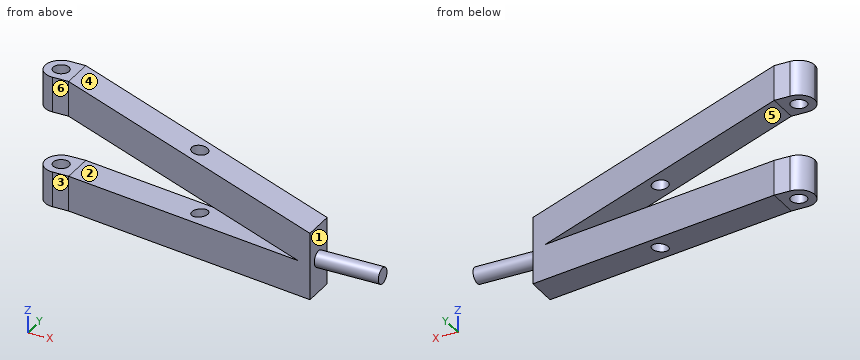
from build123d import *

# Parameters (mm, degrees)
SKETCH10_W              = 27.94
SKETCH10_H              = 25.4
SKETCH12_W              = 27.94
SKETCH12_H              = 25.4
BOSS_EXTRUDE2_DEPTH     = 25.4
SKETCH13_R              = 6.35
CUT_EXTRUDE4_DEPTH      = 105.14
CUT_EXTRUDE5_DEPTH      = 105.14
SKETCH15_R              = 6.35
BOSS_EXTRUDE3_DEPTH     = 50.8
SKETCH16_R              = 6.35
CUT_EXTRUDE6_DEPTH      = 53.07
CUT_EXTRUDE6_DEPTH_BACK = 53.07


with BuildPart() as part:
    # Sweep3: sweep along a curve in space
    with BuildLine() as sweep3_path:
        Line((12.7, 0, 38.1), (241.3, -69.85, 12.7))
    # Sketch10 → Sweep3 (sweep)
    with BuildSketch(Plane(origin=(12.7, 0, 0), x_dir=(0, 0, -1), z_dir=(1, 0, 0))):
        with Locations((-38.1, 0)):
            Rectangle(SKETCH10_W, SKETCH10_H)
    sweep3 = sweep(path=sweep3_path.line)

    # Sketch12 → Boss-Extrude2 (add)
    with BuildSketch(Plane(origin=(12.7, 0, 0), x_dir=(0, 0, -1), z_dir=(1, 0, 0))):
        with Locations((-38.1, 0)):
            Rectangle(SKETCH12_W, SKETCH12_H)
    boss_extrude2 = extrude(amount=-BOSS_EXTRUDE2_DEPTH)

    # Mirror5: Sweep3, Boss-Extrude2 across plane
    add(sweep3.mirror(Plane.XY))
    add(boss_extrude2.mirror(Plane.XY))

    # Sketch13 → Cut-Extrude4 (cut, through all)
    with BuildSketch(Plane(origin=(0, 0, -52.07), x_dir=(-1, 0, 0), z_dir=(0, 0, -1))):
        Circle(SKETCH13_R)
    extrude(amount=-CUT_EXTRUDE4_DEPTH, mode=Mode.SUBTRACT)

    # Sketch14 → Cut-Extrude5 (cut, through all)
    with BuildSketch(Plane(origin=(0, 0, -52.07), x_dir=(-1, 0, 0), z_dir=(0, 0, -1))):
        with BuildLine():
            Line((12.7, 12.7), (0, 12.7))
            ThreePointArc((0, 12.7), (8.980256121, 8.980256121), (12.7, 0))
            Line((12.7, 0), (12.7, 12.7))
        make_face()
    cut_extrude5 = extrude(amount=-CUT_EXTRUDE5_DEPTH, mode=Mode.SUBTRACT)

    # Mirror6: Cut-Extrude5 across plane
    add(cut_extrude5.mirror(Plane.ZX), mode=Mode.SUBTRACT)

    # Sketch15 → Boss-Extrude3 (add)
    with BuildSketch(Plane(origin=(241.3, 0, 0), x_dir=(0, 0, -1), z_dir=(1, 0, 0))):
        with Locations((0, -69.85)):
            Circle(SKETCH15_R)
    extrude(amount=BOSS_EXTRUDE3_DEPTH)

    # Sketch16 → Cut-Extrude6 (cut, two sides)
    with BuildSketch(Plane.XY) as cut_extrude6_sk:
        with Locations((128.524, -34.925)):
            Circle(SKETCH16_R)
    extrude(amount=CUT_EXTRUDE6_DEPTH, mode=Mode.SUBTRACT)
    extrude(cut_extrude6_sk.sketch, amount=-CUT_EXTRUDE6_DEPTH_BACK, mode=Mode.SUBTRACT)


solid = part.part
Check sheet for the modelled part. Datum: model origin and axes. Units: mm. Face numbers are marked on the shaded views. A direction names the side the tool comes from. Round coordinates to 2 decimals unless told otherwise and drop trailing zeros. Loops run counter-clockwise (first coordinate to the right, second up) from the corner with the lowest first, then second, coordinate; pieces in that order, holes last. Notation, with made-up numbers: (-30.5, -31) -> (11.5, -31) arc R23 cw to (11.5, -12) -> close; hole circle Ø8 at (19.5, 38.5). An arc over 180 degrees is marked (long way). Put each result on its own line as item: value. Start each with the question number.
1. Access from +Z, -Z, +X, -X, +Y, -Y to the whole of each face (thin tool, end or side, straight path). Record for the marked faces 1, 2 and 3.
2. Gauge pin test, flat ends, axial feed: pin 1 (16.5 mm diameter, centred on x = 128.524, y = -34.925, fed in from -Z); pin 2 (8 mm diameter, centred on x = 86.5, y = -25.5, fed in from -Z); pin 3 (10 mm diameter, centred on x = 150.5, z = -20, fed in from -Y); pin 4 (20.5 mm diameter, centred on x = 0, y = 0, fed in from -Z). Record the tip position at first contact, or that the pin passes through.
3. Scan lines: probe 1 along Y at (x, z) = (0, -30.5); probe 2 along Z at (x, y) = (139.5, -37); probe 3 along Y at (x, z) = (90, 30.5). Record each from-to range of solid material in increasing order.
4. Section check D-D (y = -69.85). Enter the section's corners in (x, z).
5. Section check A-A (y = -23.5). Enter the section's corners in (x, z), plus the area to 3 significant figures.
6. Draft check along Z on the marked faces 4, 5 and 6. Enter one of: +Z half, -Z half, draft (parallel to the pull), parting line (faces both ways), or undercut.
7. Section check B-B (x = 203.5). Enter the section's corners in (y, z), plus the area to 3 significant figures.
Findings:
1. face 1: +X
1. face 2: -X, +Y, -Y
1. face 3: +Z, -Z, -X, -Y
2. pin 1: stops at z = -40.12
2. pin 2: stops at z = -44.31
2. pin 3: stops at y = -56.33
2. pin 4: stops at z = -52.07
3. probe 1: y = -12.7 to -6.35, 6.35 to 12.7
3. probe 2: z = -37.98 to -10.04, 10.04 to 37.98
3. probe 3: y = -36.32 to -10.92
4. outline: (199.74, -31.29) -> (241.3, -26.67) -> (241.3, -6.35) -> (292.1, -6.35) -> (292.1, 6.35) -> (241.3, 6.35) -> (241.3, 26.67) -> (199.74, 31.29) -> (199.74, 3.35) -> (229.87, 0) -> (199.74, -3.35) -> close
5. outline: (48.05, -48.14) -> (131.17, -38.91) -> (131.17, -10.97) -> (48.05, -20.2) -> close; (48.05, 20.2) -> (131.17, 10.97) -> (131.17, 38.91) -> (48.05, 48.14) -> close
5. area: 4,650 mm^2
6. face 4: +Z half
6. face 5: undercut
6. face 6: draft
7. outline: (-71, -30.87) -> (-45.6, -30.87) -> (-45.6, -2.93) -> (-71, -2.93) -> close; (-71, 2.93) -> (-45.6, 2.93) -> (-45.6, 30.87) -> (-71, 30.87) -> close
7. area: 1,420 mm^2
